Answer from the drawing. Dimensions are ordinates in mm from the lowest x, y and z of the part. A direction names the side the tool comes from. Round coordinates to 2 decimals unless told otherwise and drop trailing zeros. Loops run counter-clockwise (first coordinate to the right, second up) from the corner with the lowest first, then second, coordinate; pieces in that order, holes last. Notation, with made-up numbers: (-0.5, -10.5) - (38.5, -10.5) arc R14 ccw to (38.5, 8.5) - close; hole circle Ø5 at (-2.5, 82). An arc over 180 degrees is marked (long way). One line per question, with ' | ' between items. Start each with the question number.
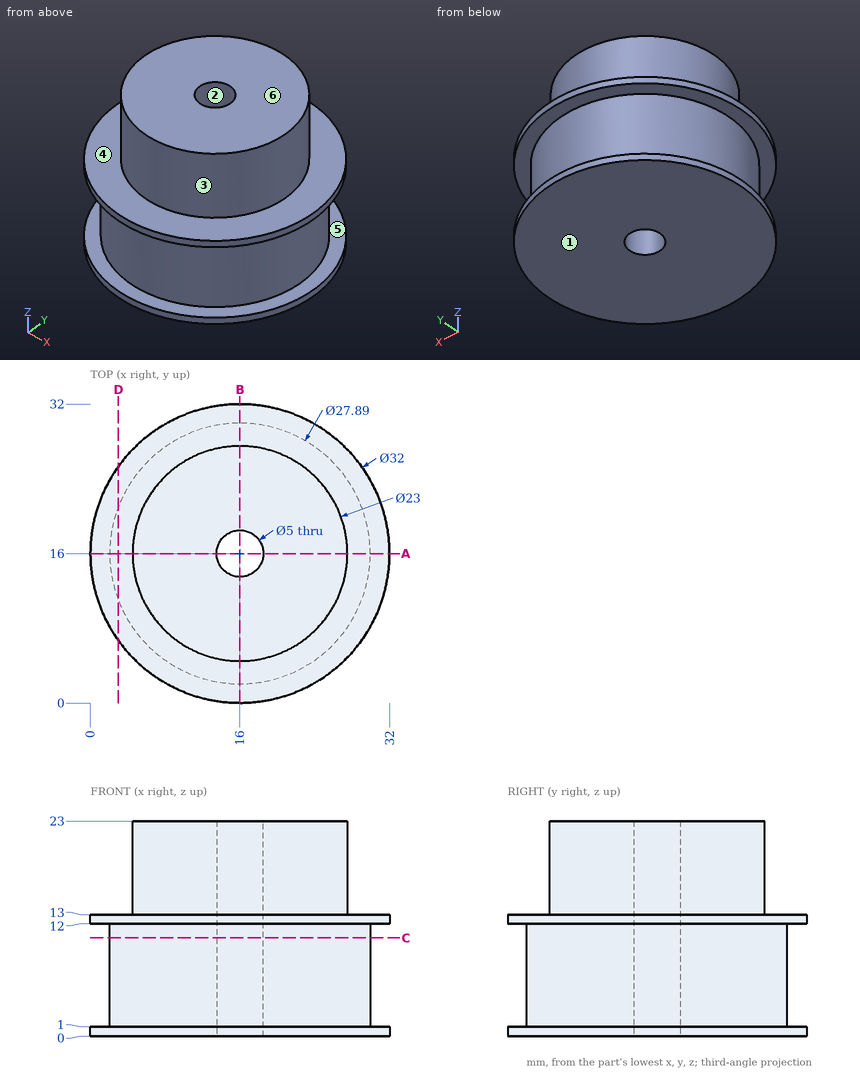
(1) A tool of negligible diameter and unlimited length cuts with its end or side. For the marked faces 4, 5 and 6, from which of +Z, -Z, +X, -X, +Y, -Y can it reach the whole face along a straight path? Write none if from no direction.
(2) Find section A-A on y = 16. Write down the section's boundary in (x, z) (3 decimals).
(3) Each of these flat-tipped pins is pushed along its axis until it touches: P1, Ø5, axis at y = 6.5, z = 14.5, coming from the +X side; P2, Ø10, axis at x = 11, z = 11, coming from the -Y side; P3, Ø4, axis at x = 7, z = 9.5, coming from the -Y side; P4, Ø5, axis at x = 27, z = 9, coming from the +Y side (3 decimals). Where does it stop, or does it pass through?
(4) Find section C-C on z = 10.5. Write down the section's boundary in (x, y) (3 decimals).
(5) Find section D-D on x = 3. Write down the section's boundary in (y, z), plus the area to 3 significant figures.
(6) Determine the mould class of the marked faces 1, 2 and 3 for opening direction Y: pulls with the +Y half, pulls with the -Y half, needs draft (parallel to the pull), parting line crosses it, or undercut.
(7) Consider L1, parallel to Z at x = 3, y = 23; L2, parallel to Y at x = 16, z = 18.25; L3, parallel to Y at x = 16, z = 11 (3 decimals). Determine where each line is inside the solid, lowest interval first.
Answer below:
1) face 4: +Z | face 5: none | face 6: +Z, +X, -X, +Y, -Y
2) outline: (0, 0) - (13.5, 0) - (13.5, 23) - (4.5, 23) - (4.5, 13) - (0, 13) - (0, 12) - (2.055, 12) - (2.055, 1) - (0, 1) - close; (18.5, 0) - (32, 0) - (32, 1) - (29.945, 1) - (29.945, 12) - (32, 12) - (32, 13) - (27.5, 13) - (27.5, 23) - (18.5, 23) - close
3) P1: x = 30.13 | P2: y = 0 | P3: y = 3.94 | P4: y = 27.055
4) outline: circle Ø27.89 at (16, 16); hole circle Ø5 at (16, 16)
5) outline: (6.67, 0) - (25.33, 0) - (25.33, 1) - (21.05, 1) - (21.05, 12) - (25.33, 12) - (25.33, 13) - (6.67, 13) - (6.67, 12) - (10.95, 12) - (10.95, 1) - (6.67, 1) - close | area: 148 mm2
6) face 1: needs draft | face 2: undercut | face 3: parting line crosses it
7) L1: 0 to 1, 12 to 13 | L2: 4.5 to 13.5, 18.5 to 27.5 | L3: 2.055 to 13.5, 18.5 to 29.945
